```python
from build123d import *

# Parameters (mm, degrees)
SKETCH1_R           = 4
BOSS_EXTRUDE1_DEPTH = 33.2
SKETCH2_R           = 3
BOSS_EXTRUDE2_DEPTH = 8
CHAMFER1_SIZE       = 0.3


with BuildPart() as part:
    # Sketch1 → Boss-Extrude1 (new, symmetric)
    with BuildSketch(Plane.XY):
        with Locations(Location((0, 0, 0), (0, 0, 180))):
            Circle(SKETCH1_R)
    extrude(amount=BOSS_EXTRUDE1_DEPTH, both=True)

    # Sketch2 → Boss-Extrude2 (add)
    with BuildSketch(Plane.XY.offset(33.2)):
        Circle(SKETCH2_R)
    boss_extrude2 = extrude(amount=BOSS_EXTRUDE2_DEPTH)

    # Mirror1: Boss-Extrude2 across plane
    add(boss_extrude2.mirror(Plane.XY))

    # Chamfer1
    chamfer1_edges = [part.edges().sort_by_distance(p)[0] for p in [
        (-3, 0, -41.2),
        (4, 0, -33.2),
        (4, 0, 33.2),
        (-3, 0, 41.2),
    ]]
    chamfer(chamfer1_edges, length=CHAMFER1_SIZE)


solid = part.part
```
Verification items for the finished model (mm, model axes). A direction names the side the tool comes from. Round coordinates to 2 decimals unless told otherwise and drop trailing zeros. Order: outer loops, then holes, each group sorted by start corner. A loop starts at its lowest first (then second) coordinate and runs counter-clockwise, first axis right, second up.
1) Material ranges on line 1 (Z direction, x = 2.75, y = -2.5); line 2 (Y direction, x = 1.5, z = 20); line 3 (Y direction, x = -0.25, z = 3.5), recorded low to high.
Geometry says:
line 1: z = -33.18 to 33.18
line 2: y = -3.71 to 3.71
line 3: y = -3.99 to 3.99
2) Cross-section at A-A, the plane x = 0. Record the cut outline in (y, z), plus the area to 3 significant figures.
Geometry says:
outline: (-4, -32.9) - (-3.7, -33.2) - (-3, -33.2) - (-3, -40.9) - (-2.7, -41.2) - (2.7, -41.2) - (3, -40.9) - (3, -33.2) - (3.7, -33.2) - (4, -32.9) - (4, 32.9) - (3.7, 33.2) - (3, 33.2) - (3, 40.9) - (2.7, 41.2) - (-2.7, 41.2) - (-3, 40.9) - (-3, 33.2) - (-3.7, 33.2) - (-4, 32.9) - close
area: 627 mm2
3) Draft check along Y on faces 1 (the flat face through (0, 0, 41.2)), 2 (the cylindrical face through (-3, 0, 37)). Enter one of: +Y half, -Y half, draft (parallel to the pull), parting line (faces both ways), or undercut.
Geometry says:
face 1: draft
face 2: parting line
4) Tool access check on faces 3 (the flat face through (1, -3, -33.2)), 4 (the flat face through (1, -3, 33.2)), 5 (the cylindrical face through (0.867, 3.905, 0.461)). Record the directions out of +Z, -Z, +X, -X, +Y, -Y that give a thin tool (end or side, any length) a straight path to the whole face; none if there is none.
Geometry says:
face 3: -Z
face 4: +Z
face 5: +Z, -Z
5) Depth check by flat-ended pin: pin 1 (1.5 mm diameter, centred on x = -2.5, z = -7, fed in from -Y). Enter the tip coordinate at first touch or a pass-through.
Geometry says:
pin 1: stops at y = -3.6
6) Cross-section at C-C, the plane z = -15.5. Record the cut outline in (x, y), plus the area to 3 significant figures.
Geometry says:
outline: circle Ø8 at (0, 0)
area: 50.3 mm2
7) Cross-section at D-D, the plane z = -34. Record the cut outline in (x, y), plus the area to 3 significant figures.
Geometry says:
outline: circle Ø6 at (0, 0)
area: 28.3 mm2
